from build123d import *

# Parameters (mm, degrees)
SKETCH_1_W             = 120
SKETCH_1_H             = 178
EXTRUDE_1_DEPTH        = 10
SKETCH_2_W             = 15
SKETCH_2_H             = 178
EXTRUDE_2_DEPTH        = 17
SKETCH_3_W             = 70
SKETCH_3_H             = 24
CUT_EXTRUDE_1_DEPTH    = 5
HOLE_WIZARD_M4_1_D     = 3.3
PATTERN_LINEAR_1_COUNT = 3
PATTERN_LINEAR_1_PITCH = 60
HOLE_WIZARD_M4_2_D     = 3.3
HOLE_WIZARD_M8_1_D     = 6.8
HOLE_WIZARD_M4_7_D     = 3.3
HOLE_WIZARD_M4_3_D     = 3.3
HOLE_WIZARD_M4_5_D     = 3.3
HOLE_WIZARD_M4_6_D     = 3.3


with BuildPart() as part:
    # 草图1 → 凸台-拉伸1 (new body)
    with BuildSketch(Plane(origin=(0, 0, 0), x_dir=(0, 0, -1), z_dir=(1, 0, 0))):
        with Locations((60, 89)):
            Rectangle(SKETCH_1_W, SKETCH_1_H)
    extrude(amount=EXTRUDE_1_DEPTH)

    # 草图2 → 凸台-拉伸2 (add)
    with BuildSketch(Plane.ZY):
        with Locations((-112.5, 89)):
            Rectangle(SKETCH_2_W, SKETCH_2_H)
        with Locations((-7.5, 89)):
            Rectangle(SKETCH_2_W, SKETCH_2_H)
    extrude(amount=EXTRUDE_2_DEPTH)

    # 草图3 → 切除-拉伸1 (cut)
    with BuildSketch(Plane.ZY):
        with Locations((-60, 115)):
            Rectangle(SKETCH_3_W, SKETCH_3_H)
    extrude(amount=-CUT_EXTRUDE_1_DEPTH, mode=Mode.SUBTRACT)

    # M4 螺纹孔1 (through all)
    with Locations(Plane(origin=(-17, 149, -112.5), x_dir=(0, 0, -1), z_dir=(-1, 0, 0))):
        with Locations((0, 0), (-105, 0)):
            hole_wizard_m4_1 = Hole(HOLE_WIZARD_M4_1_D / 2)

    # 阵列(线性)1: M4 螺纹孔1 ×3
    with Locations(*[(0, -i * PATTERN_LINEAR_1_PITCH, 0) for i in range(1, PATTERN_LINEAR_1_COUNT)]):
        add(hole_wizard_m4_1, mode=Mode.SUBTRACT)

    # M4 螺纹孔2 (through all)
    with Locations(Plane(origin=(0, 173, -89.5), x_dir=(0, 0, -1), z_dir=(-1, 0, 0))):
        with Locations((0, 0), (-59, 0), (-11.5, 168), (-47.5, 168)):
            Hole(HOLE_WIZARD_M4_2_D / 2)

    # M8 螺纹孔1 (through all)
    with Locations(Plane(origin=(0, 115, -86), x_dir=(0, 0, -1), z_dir=(-1, 0, 0))):
        with Locations((0, 0), (-52, 0)):
            Hole(HOLE_WIZARD_M8_1_D / 2)

    # M4 螺纹孔7 (through all)
    with Locations(Plane(origin=(0, 115, -69), x_dir=(0, 0, -1), z_dir=(-1, 0, 0))):
        with Locations((0, 0), (-18, 0), (0, -9), (-18, -9)):
            Hole(HOLE_WIZARD_M4_7_D / 2)

    # M4 螺纹孔3 (through all)
    with Locations(Plane(origin=(0, 63, -69), x_dir=(0, 0, -1), z_dir=(-1, 0, 0))):
        with Locations((0, 0), (-18, 0), (0, 9), (-18, 9)):
            Hole(HOLE_WIZARD_M4_3_D / 2)

    # M4 螺纹孔5 (through all)
    with Locations(Plane(origin=(0, 162, -72.5), x_dir=(0, 0, -1), z_dir=(-1, 0, 0))):
        with Locations((0, 0), (-26, 0), (0, 146), (-26, 146), (-26, 120), (0, 120)):
            Hole(HOLE_WIZARD_M4_5_D / 2)

    # M4 螺纹孔6 (through all)
    with Locations(Plane(origin=(0, 136, -72.5), x_dir=(0, 0, -1), z_dir=(-1, 0, 0))):
        with Locations((0, 0), (-26, 0)):
            Hole(HOLE_WIZARD_M4_6_D / 2)


solid = part.part
Here's how the part is built. I have some questions about the finished solid (model axes, mm). A direction names the side the tool comes from. Give positions to 0.01 mm unless a question says otherwise; leave off trailing zeros. Order: outer loops, then holes, each group sorted by start corner. A loop starts at its lowest first (then second) coordinate and runs counter-clockwise, first axis right, second up. Notation, with made-up numbers: (-13, -13.5) -> (14, -13.5) arc R19 cw to (14, 22.5) -> close; hole circle Ø11 at (84.25, -2.5). An arc over 180 degrees is marked (long way). Use a Markdown table: item, result. Add a question column.
Item 1: Imagine slicing it at D-D on z = -100.5. Please give me the cut outline in (x, y), plus the area to 3 significant figures.
Item 2: I need wall thicknesses on line 1 (Z direction, x = 6, y = 115); line 2 (Y direction, x = 6, z = -72.5); line 3 (Y direction, x = -5.25, z = -7.5). Which ranges of each line are inside material? Lowest first, please.
Item 3: Will this pin go through, and if not, where does the flat tip stop? pin 1 (4.5 mm diameter, centred on y = 42, z = -46.5, fed in from -X).
Item 4: If we mould it in two halves opening along Y, with no side actions, what happens to faces 4 (the face through (7.5, 125.6, -69.4)), 5 (the face through (3, 0, -61)), 6 (the face through (-8, 88, -15))? For each: pulls with the +Y half, pulls with the -Y half, needs draft (parallel to the pull), parting line crosses it, or undercut.
Item 5: For faces 1 (the face through (2, 127, -60)), 2 (the face through (7.5, 116.6, -69.4)), 3 (the face through (-8, 88, -105)), which set-ups out of +Z, -Z, +X, -X, +Y, -Y let a thin tool reach every point of the face, with its end or its side?
Item 6: Imagine slicing it at B-B on x = 3. Give the number of separate pieces and of enclosed holes in the cut face, plus the area to 3 significant figures.
Item 7: Imagine slicing it at C-C on y = 107. Please give me the cut outline in (x, z).
Item 8: Imagine slicing it at A-A on x = -14. Please give me the cut outline in (y, z), plus the area to 3 significant figures.
Data:
| question | item | result |
|---|---|---|
| 1 | outline | (0, 0) -> (10, 0) -> (10, 178) -> (0, 178) -> close |
| 1 | area | 1,780 mm² |
| 2 | line 1 | z = -120 to -89.4, -82.6 to -70.65, -67.35 to -52.65, -49.35 to -37.4, -30.6 to 0 |
| 2 | line 2 | y = 0 to 14.35, 17.65 to 40.35, 43.65 to 134.35, 137.65 to 160.35, 163.65 to 178 |
| 2 | line 3 | y = 0 to 27.35, 30.65 to 87.35, 90.65 to 147.35, 150.65 to 178 |
| 3 | pin 1 | stops at x = 0 |
| 4 | face 4 | undercut |
| 4 | face 5 | pulls with the -Y half |
| 4 | face 6 | needs draft |
| 5 | face 1 | -X |
| 5 | face 2 | +X, -X |
| 5 | face 3 | -X, +Y, -Y |
| 6 | separate pieces | 1 |
| 6 | enclosed holes | 23 |
| 6 | area | 19,500 mm² |
| 7 | outline | (-17, -120) -> (10, -120) -> (10, 0) -> (-17, 0) -> (-17, -15) -> (0, -15) -> (0, -25) -> (5, -25) -> (5, -95) -> (0, -95) -> (0, -105) -> (-17, -105) -> close |
| 8 | outline | (0, -120) -> (178, -120) -> (178, -105) -> (0, -105) -> close; (0, -15) -> (178, -15) -> (178, 0) -> (0, 0) -> close; hole circle Ø3.3 at (29, -112.5); hole circle Ø3.3 at (29, -7.5); hole circle Ø3.3 at (89, -112.5); hole circle Ø3.3 at (89, -7.5); hole circle Ø3.3 at (149, -112.5); hole circle Ø3.3 at (149, -7.5) |
| 8 | area | 5,290 mm² |
